Can you work these out from the model? Positions are in its coordinate system, mm. Face numbers are marked on the shaded views. A direction names the side the tool comes from. Give positions to 0.01 mm unless a question says otherwise; leave off trailing zeros. Loops run counter-clockwise (first coordinate to the right, second up) from the corner with the lowest first, then second, coordinate; pieces in that order, holes last. Notation, with made-up numbers: (20, -7.75) - (52, -7.75) arc R27 cw to (52, 21.25) - close; hole circle Ø7 at (-38, 12). An arc over 180 degrees is marked (long way). Answer as a JSON object with one key per item and string values. Group by question number.
Item 1: Thinking about a two-plate mould opening in X: for the marked faces 4, 5, 6 and 7, which applies, pulls with the +X half, pulls with the -X half, needs draft (parallel to the pull), parting line crosses it, or undercut?
Item 2: Please list where these lines run through material, in increasing order: L1, parallel to Y at x = -24.48, z = 2.25; L2, parallel to Y at x = -25, z = 6; L3, parallel to Z at x = -26, y = 7.5.
Item 3: Will these pins go through, and if not, where does the flat tip stop? pin 1 (5.5 mm diameter, centred on x = 0.5, z = -43.5, fed in from -Y); pin 2 (6 mm diameter, centred on x = -9, z = -34.5, fed in from -Y); pin 3 (2 mm diameter, centred on y = -11, z = -37.5, fed in from +X) (3 decimals).
Item 4: Suppose I cut it at B-B on z = -32. Write out the boundary of the cut face in (x, y) (3 decimals).
Item 5: Which directions (+Z, -Z, +X, -X, +Y, -Y) give clear straight access to the entire face, cutting with the end or side of a thin tool? Please do the marked faces 1, 2 and 3.
Item 6: Suppose I cut it at D-D on y = 24.48. Write out the boundary of the cut face in (x, z), and give its area (3 significant figures).
Item 7: Suppose I cut it at A-A on x = 25.5. Write out the boundary of the cut face in (y, z).
Item 8: Suppose I cut it at C-C on y = 3. Write out the boundary of the cut face in (x, z).
from build123d import *

# Parameters (mm, degrees)
CROQUIS2_W              = 75
CROQUIS2_H              = 75
SALIENTE_EXTRUIR1_DEPTH = 10
SALIENTE_EXTRUIR2_DEPTH = 100
CHAFL_N1_SIZE           = 25
CHAFL_N1_SIZE_2         = 15
CHAFL_N2_SIZE           = 25
CHAFL_N2_SIZE_2         = 15
CORTAR_EXTRUIR1_REACH   = 112.598
CHAFL_N3_SIZE           = 5
REDONDEO1_R             = 6
REDONDEO2_R             = 20
SKETCH1_R               = 7.65
SKETCH1_R_2             = 6
CUT_EXTRUDE2_DEPTH      = 10


with BuildPart() as part:
    # Croquis2 → Saliente-Extruir1 (new body)
    with BuildSketch(Plane(origin=(0, 0, 0), x_dir=(0, 1, 0), z_dir=(0, 0, 1))):
        Rectangle(CROQUIS2_W, CROQUIS2_H)
    extrude(amount=SALIENTE_EXTRUIR1_DEPTH)

    # Croquis2<3> → Saliente-Extruir2 (add)
    with BuildSketch(Plane(origin=(0, 0, 0), x_dir=(0, 1, 0), z_dir=(0, 0, 1))):
        with BuildLine():
            Line((-21.5, 9.375), (-21.5, -9.375))
            Line((-21.5, -9.375), (-8.267972847, -9.375))
            ThreePointArc((-8.267972847, -9.375), (-12.5, 0), (-8.267972847, 9.375))
            Line((-8.267972847, 9.375), (-21.5, 9.375))
        make_face()
        with BuildLine():
            ThreePointArc((8.267972847, 9.375), (12.5, 0), (8.267972847, -9.375))
            Line((8.267972847, -9.375), (21.5, -9.375))
            Line((21.5, -9.375), (21.5, 9.375))
            Line((21.5, 9.375), (8.267972847, 9.375))
        make_face()
    extrude(amount=-SALIENTE_EXTRUIR2_DEPTH)

    # Chaflán1
    # the kernel refuses this chamfer: 25, 15 mm, written as the material it takes off along each edge
    with BuildSketch(Plane(origin=(74.03152743, 21.5, -100), x_dir=(0, 0.01989341895858247, 0.9998021063601227), z_dir=(-1, 0, 0))) as chafl_n1_piece_1:
        Polygon((CHAFL_N1_SIZE * 0.99980210636, -CHAFL_N1_SIZE * 0.0198934189586), (-CHAFL_N1_SIZE_2 * 0.0198934189586, -CHAFL_N1_SIZE_2 * 0.99980210636), (0, 0), align=None)
    extrude(amount=148.06305486, mode=Mode.SUBTRACT)

    # Chaflán2
    # the kernel refuses this chamfer: 25, 15 mm, written as the material it takes off along each edge
    with BuildSketch(Plane(origin=(-74.03152743, -21.5, -100), x_dir=(0, -0.01989341895858247, 0.9998021063601227), z_dir=(1, 0, 0))) as chafl_n2_piece_1:
        Polygon((CHAFL_N2_SIZE * 0.99980210636, -CHAFL_N2_SIZE * 0.0198934189586), (-CHAFL_N2_SIZE_2 * 0.0198934189586, -CHAFL_N2_SIZE_2 * 0.99980210636), (0, 0), align=None)
    extrude(amount=148.06305486, mode=Mode.SUBTRACT)

    # Croquis2<4> → Cortar-Extruir1 (cut, up to next)
    with BuildSketch(Plane(origin=(0, 0, 0), x_dir=(0, 1, 0), z_dir=(0, 0, 1)), mode=Mode.PRIVATE) as cortar_extruir1_sk1:
        with BuildLine():
            ThreePointArc((-8.267972847, 9.375), (-12.5, 0), (-8.267972847, -9.375))
            Line((-8.267972847, -9.375), (8.267972847, -9.375))
            ThreePointArc((8.267972847, -9.375), (11.392972847, -5.142972847), (12.5, 0))
            ThreePointArc((12.5, 0), (11.392972847, 5.142972847), (8.267972847, 9.375))
            Line((8.267972847, 9.375), (-8.267972847, 9.375))
        make_face()
    cortar_extruir1_tool1 = extrude(cortar_extruir1_sk1.sketch, amount=CORTAR_EXTRUIR1_REACH, mode=Mode.PRIVATE) & part.part
    # Croquis2<4> → Cortar-Extruir1 (cut, up to next)
    with BuildSketch(Plane(origin=(0, 0, 0), x_dir=(0, 1, 0), z_dir=(0, 0, 1)), mode=Mode.PRIVATE) as cortar_extruir1_sk2:
        with BuildLine():
            Line((8.267972847, -9.375), (-8.267972847, -9.375))
            ThreePointArc((-8.267972847, -9.375), (0, -12.5), (8.267972847, -9.375))
        make_face()
    cortar_extruir1_tool2 = extrude(cortar_extruir1_sk2.sketch, amount=CORTAR_EXTRUIR1_REACH, mode=Mode.PRIVATE) & part.part
    # Croquis2<4> → Cortar-Extruir1 (cut, up to next)
    with BuildSketch(Plane(origin=(0, 0, 0), x_dir=(0, 1, 0), z_dir=(0, 0, 1)), mode=Mode.PRIVATE) as cortar_extruir1_sk3:
        with BuildLine():
            ThreePointArc((8.267972847, 9.375), (0, 12.5), (-8.267972847, 9.375))
            Line((-8.267972847, 9.375), (8.267972847, 9.375))
        make_face()
    cortar_extruir1_tool3 = extrude(cortar_extruir1_sk3.sketch, amount=CORTAR_EXTRUIR1_REACH, mode=Mode.PRIVATE) & part.part
    add(cortar_extruir1_tool1.solids().sort_by_distance((0, 0, 0))[0], mode=Mode.SUBTRACT)
    add(cortar_extruir1_tool2.solids().sort_by_distance((10.639442, 0, 0))[0], mode=Mode.SUBTRACT)
    add(cortar_extruir1_tool3.solids().sort_by_distance((-10.639442, 0, 0))[0], mode=Mode.SUBTRACT)

    # Chaflán3
    chafl_n3_edges = [part.edges().sort_by_distance(p)[0] for p in [
        (0, 21.5, -75),
        (0, -21.5, -75),
    ]]
    chamfer(chafl_n3_edges, length=CHAFL_N3_SIZE)

    # Redondeo1
    redondeo1_edges = [part.edges().sort_by_distance(p)[0] for p in [
        (-9.375, -21.5, -35),
        (9.375, -21.5, -35),
        (9.375, 21.5, -35),
        (-9.375, 21.5, -35),
    ]]
    fillet(redondeo1_edges, radius=REDONDEO1_R)

    # Redondeo2
    redondeo2_edges = [part.edges().sort_by_distance(p)[0] for p in [
        (37.5, -37.5, 5),
        (-37.5, -37.5, 5),
        (-37.5, 37.5, 5),
        (37.5, 37.5, 5),
    ]]
    fillet(redondeo2_edges, radius=REDONDEO2_R)

    # Sketch1 → Cut-Extrude2 (cut)
    with BuildSketch(Plane.XY.offset(10)):
        with Locations((25.5, 19.5)):
            Circle(SKETCH1_R)
        with Locations((-24.48, 24.48)):
            Circle(SKETCH1_R_2)
        with Locations((-25.5, -19.5)):
            Circle(SKETCH1_R)
        with Locations((24.48, -24.48)):
            Circle(SKETCH1_R_2)
    extrude(amount=-CUT_EXTRUDE2_DEPTH, mode=Mode.SUBTRACT)


solid = part.part
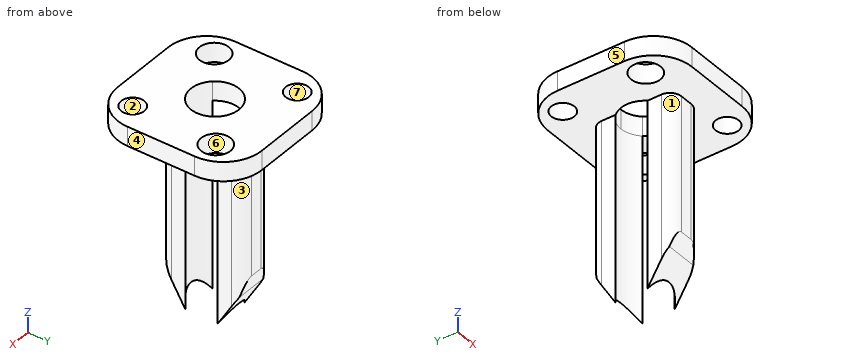
Worked out:
{
 "1": {"face 4": "pulls with the +X half", "face 5": "pulls with the -X half", "face 6": "undercut", "face 7": "undercut"},
 "2": {"L1": "y = -36.24 to -27.08, -11.92 to 18.48, 30.48 to 36.24", "L2": "y = -36.04 to -27.13, -11.87 to 18.5, 30.46 to 36.04", "L3": "z = 0 to 10"},
 "3": {"pin 1": "stops at y = -21.5", "pin 2": "stops at y = -20.9", "pin 3": "stops at x = 9.375"},
 "4": {"outline": "(-9.375, -15.5) arc R6 ccw to (-3.375, -21.5) - (3.375, -21.5) arc R6 ccw to (9.375, -15.5) - (9.375, -8.268) arc R12.5 cw to (-9.375, -8.268) - close; (-9.375, 8.268) arc R12.5 cw to (9.375, 8.268) - (9.375, 15.5) arc R6 ccw to (3.375, 21.5) - (-3.375, 21.5) arc R6 ccw to (-9.375, 15.5) - close"},
 "5": {"face 1": "-Z, -X, -Y", "face 2": "+Z, -Z", "face 3": "-Z, +X, +Y"},
 "6": {"outline": "(-36.24, 0) - (-30.48, 0) - (-30.48, 10) - (-36.24, 10) - close; (-18.48, 0) - (19.69, 0) - (19.69, 10) - (-18.48, 10) - close; (31.31, 0) - (36.24, 0) - (36.24, 10) - (31.31, 10) - close", "area": "489 mm2"},
 "7": {"outline": "(-35.83, 0) - (-30.39, 0) - (-30.39, 10) - (-35.83, 10) - close; (-18.57, 0) - (11.85, 0) - (11.85, 10) - (-18.57, 10) - close; (27.15, 0) - (35.83, 0) - (35.83, 10) - (27.15, 10) - close"},
 "8": {"outline": "(-37.5, 0) - (-12.13, 0) - (-12.13, 10) - (-37.5, 10) - close; (12.13, 0) - (37.5, 0) - (37.5, 10) - (12.13, 10) - close"}
}
